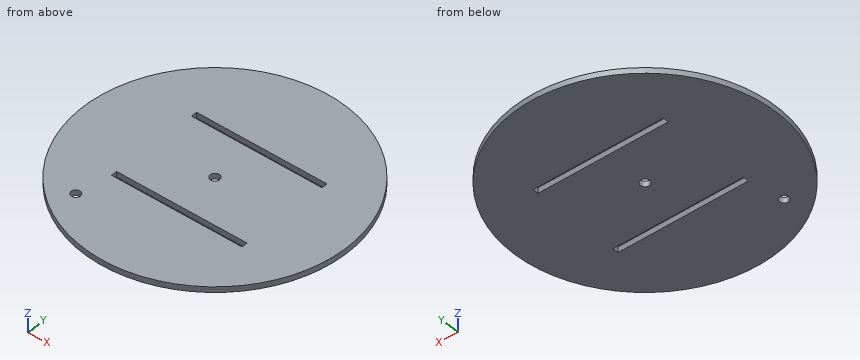
from build123d import *

# Parameters (mm, degrees)
F0_R     = 75
F0_R_2   = 2.6
F0_W     = 75
F0_H     = 3.4
F0_R_3   = 2.7
F1_DEPTH = 3.2


with BuildPart() as f1:
    # F0 (on Top) → F1 (new body)
    with BuildSketch(Plane.XY):
        Circle(F0_R)
        with Locations((-38.605813, -48.087154)):
            Circle(F0_R_2, mode=Mode.SUBTRACT)
        with Locations((2.5, -26.7)):
            Rectangle(F0_W, F0_H, mode=Mode.SUBTRACT)
        Circle(F0_R_3, mode=Mode.SUBTRACT)
        with Locations((2.5, 26.7)):
            Rectangle(F0_W, F0_H, mode=Mode.SUBTRACT)
    extrude(amount=F1_DEPTH)


solid = f1.part
Here's how the part is built. I have some questions about the finished solid (model axes, mm). Coordinates: 2 decimals unless noted, no trailing zeros. Order: outer loops, then holes, each group sorted by start corner. A loop starts at its lowest first (then second) coordinate and runs counter-clockwise, first axis right, second up. Notation, with made-up numbers: (80.25, 14) - (93.25, 14) arc R32 ccw to (93.25, 53) - close; hole circle Ø9 at (30, 59). An arc over 180 degrees is marked (long way). Use CSV: the item, a comma, the result in double quotes. Start each with the question number.
1. Suppose I cut it at C-C on z = 1.5. List the corners of the cut face in (x, y) for me, then the cut area to 3 significant figures.
2. Suppose I cut it at A-A on x = 0. List the corners of the cut face in (y, z) for me.
3. Suppose I cut it at D-D on x = 31. List the corners of the cut face in (y, z) for me.
4. Suppose I cut it at B-B on y = 0. List the corners of the cut face in (x, z) for me.
5. Please list where these lines run through material, in increasing order: line 1 (Y direction, x = 0, z = 1.75); line 2 (Y direction, x = 4, z = 1.7); line 3 (Y direction, x = -28, z = 0.8). Write a range as from..to.
6. I'm going to push flat-ended pins straight in: pin 1 (1.5 mm diameter, centred on x = 23.5, z = 1, fed in from +Y); pin 2 (1.5 mm diameter, centred on y = 60, z = 2, fed in from +X); pin 3 (1.6 mm diameter, centred on y = -26, z = 2, fed in from -X). Where does each tip first touch, or does it pass through?
Output:
1,outline,"circle Ø150 at (0, 0); hole circle Ø5.2 at (-38.61, -48.09); hole (-35, -28.4) - (40, -28.4) - (40, -25) - (-35, -25) - close; hole (-35, 25) - (40, 25) - (40, 28.4) - (-35, 28.4) - close; hole circle Ø5.4 at (0, 0)"
1,area,"17,100 mm2"
2,outline,"(-75, 0) - (-28.4, 0) - (-28.4, 3.2) - (-75, 3.2) - close; (-25, 0) - (-2.7, 0) - (-2.7, 3.2) - (-25, 3.2) - close; (2.7, 0) - (25, 0) - (25, 3.2) - (2.7, 3.2) - close; (28.4, 0) - (75, 0) - (75, 3.2) - (28.4, 3.2) - close"
3,outline,"(-68.29, 0) - (-28.4, 0) - (-28.4, 3.2) - (-68.29, 3.2) - close; (-25, 0) - (25, 0) - (25, 3.2) - (-25, 3.2) - close; (28.4, 0) - (68.29, 0) - (68.29, 3.2) - (28.4, 3.2) - close"
4,outline,"(-75, 0) - (-2.7, 0) - (-2.7, 3.2) - (-75, 3.2) - close; (2.7, 0) - (75, 0) - (75, 3.2) - (2.7, 3.2) - close"
5,line 1,"y = -75..-28.4, -25..-2.7, 2.7..25, 28.4..75"
5,line 2,"y = -74.89..-28.4, -25..25, 28.4..74.89"
5,line 3,"y = -69.58..-28.4, -25..25, 28.4..69.58"
6,pin 1,"stops at y = 71.47"
6,pin 2,"stops at x = 45.98"
6,pin 3,"stops at x = -70.64"
